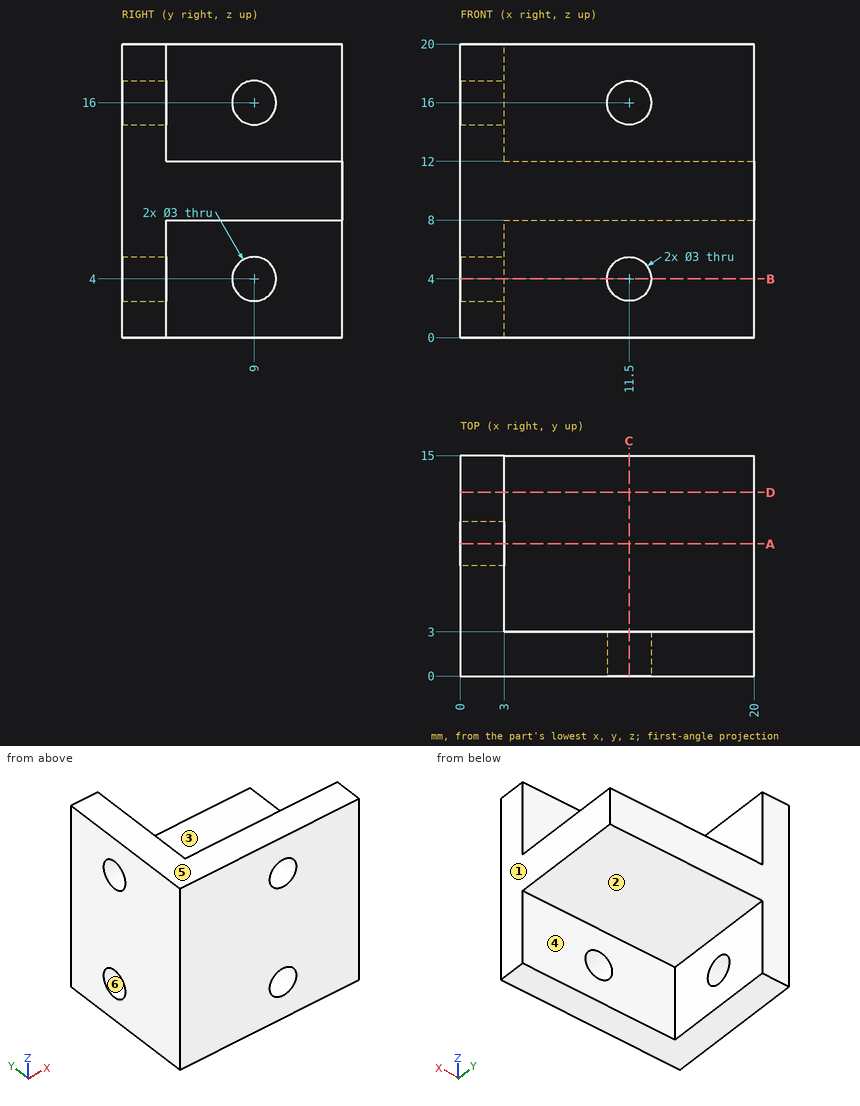
Here's the drawing with two shaded views (mm, measured from the low corner). I have some questions. A direction names the side the tool comes from. Round coordinates to 2 decimals unless told otherwise and drop trailing zeros. Order: outer loops, then holes, each group sorted by start corner. A loop starts at its lowest first (then second) coordinate and runs counter-clockwise, first axis right, second up. Notation, with made-up numbers: (29, 11) -> (46, 11) arc R24 ccw to (46, 47) -> close; hole circle Ø1 at (10, -17). An arc over 180 degrees is marked (long way). Return JSON: item names as keys, results as strings.
Q1. If we section it at D-D on y = 12.5: List the corners of the cut face in (x, z) for me.
Filled sheet:
{"outline": "(0, 0) -> (3, 0) -> (3, 8) -> (20, 8) -> (20, 12) -> (3, 12) -> (3, 20) -> (0, 20) -> close"}
Q2. Which directions (+Z, -Z, +X, -X, +Y, -Y) give clear straight access to the entire face, cutting with the end or side of a thin tool? Please do the marked faces 1, 2 and 3.
Filled sheet:
{"face 1": "+Z, -Z, +X, +Y, -Y", "face 2": "-Z, +X, +Y", "face 3": "+Z, +X, +Y"}
Q3. If we section it at A-A on y = 9: List the corners of the cut face in (x, z) for me.
Filled sheet:
{"outline": "(0, 0) -> (3, 0) -> (3, 2.5) -> (0, 2.5) -> close; (0, 5.5) -> (3, 5.5) -> (3, 8) -> (20, 8) -> (20, 12) -> (3, 12) -> (3, 14.5) -> (0, 14.5) -> close; (0, 17.5) -> (3, 17.5) -> (3, 20) -> (0, 20) -> close"}
Q4. I need wall thicknesses on line 1 along Z through (x, y) = (11.5, 2.4); line 2 along Y through (x, z) = (1.1, 4); line 3 along X through (y, z) = (2.25, 4). Which ranges of each line are inside material? Lowest first, please. Write a range as from..to.
Filled sheet:
{"line 1": "z = 0..2.5, 5.5..14.5, 17.5..20", "line 2": "y = 0..7.5, 10.5..15", "line 3": "x = 0..10, 13..20"}
Q5. If we mould it in two halves opening along Z, with no side actions, what happens to the marked faces 4, 5 and 6? For each: released by +Z, released by -Z, zero draft, split by the parting line, or undercut.
Filled sheet:
{"face 4": "zero draft", "face 5": "released by +Z", "face 6": "undercut"}
Q6. For pin 1 Ø2.5 at (y, z) = (7, 4) entering from +X; pin 2 Ø1 at (x, y) = (7, 10.5) entering from +Z; pin 3 Ø4 at (x, z) = (11.5, 16) entering from +Y; pin 4 Ø2.5 at (y, z) = (9, 16) entering from +X, each with a flat end and sliding along its axis, tell me the tip position at first contact or that it passes through.
Filled sheet:
{"pin 1": "stops at x = 3", "pin 2": "stops at z = 12", "pin 3": "stops at y = 3", "pin 4": "passes through"}
Q7. If we section it at C-C on x = 11.5: List the corners of the cut face in (y, z) for me.
Filled sheet:
{"outline": "(0, 0) -> (3, 0) -> (3, 2.5) -> (0, 2.5) -> close; (0, 5.5) -> (3, 5.5) -> (3, 8) -> (15, 8) -> (15, 12) -> (3, 12) -> (3, 14.5) -> (0, 14.5) -> close; (0, 17.5) -> (3, 17.5) -> (3, 20) -> (0, 20) -> close"}
Q8. If we section it at B-B on z = 4: List the corners of the cut face in (x, y) for me, plus the area to 3 significant figures.
Filled sheet:
{"outline": "(0, 0) -> (10, 0) -> (10, 3) -> (3, 3) -> (3, 7.5) -> (0, 7.5) -> close; (0, 10.5) -> (3, 10.5) -> (3, 15) -> (0, 15) -> close; (13, 0) -> (20, 0) -> (20, 3) -> (13, 3) -> close", "area": "78.0 mm^2"}
